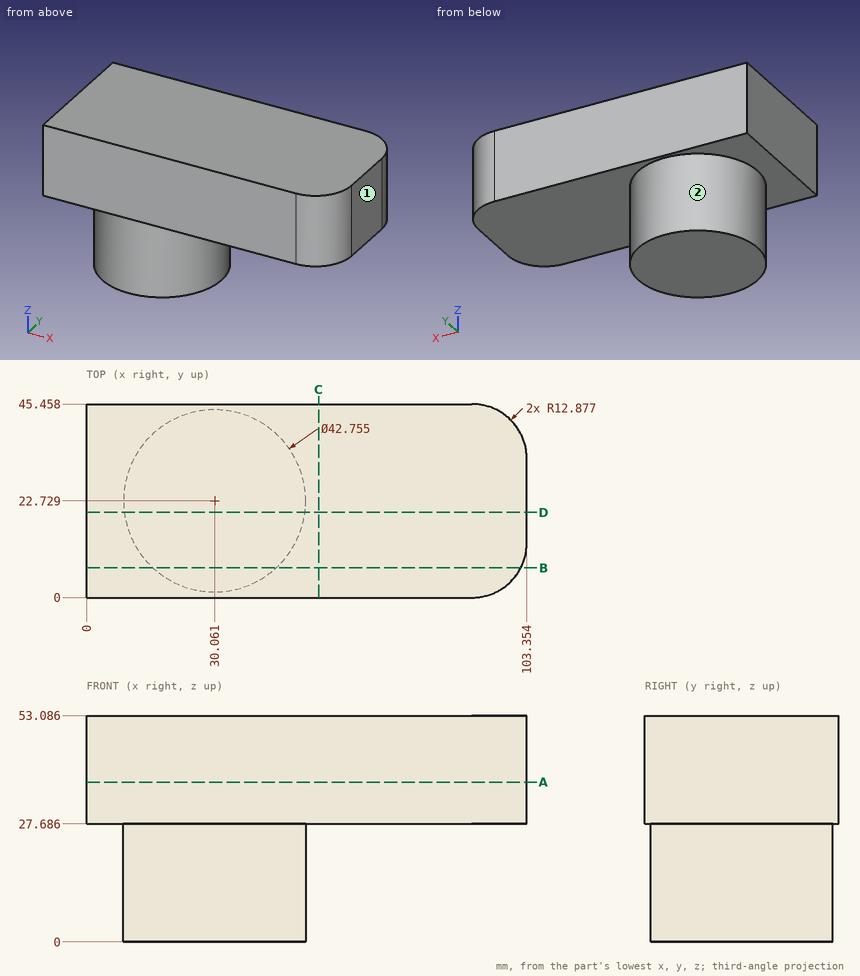
Here's the drawing with two shaded views (mm, measured from the low corner). I have some questions. A direction names the side the tool comes from. Give positions to 0.01 mm unless a question says otherwise; leave off trailing zeros. Loops run counter-clockwise (first coordinate to the right, second up) from the corner with the lowest first, then second, coordinate; pieces in that order, holes last. Notation, with made-up numbers: M 21,29 L 78,29 A16 cw 78,52 Z; hole C 52,83.25 d11. An arc over 180 degrees is marked long. Answer in a Markdown table with one row per item.
1. Suppose I cut it at C-C on x = 54.5. Write out the boundary of the cut face in (y, z).
Taken from the geometry:
| item | result |
|---|---|
| outline | M 0,27.69 L 45.46,27.69 L 45.46,53.09 L 0,53.09 Z |
2. Suppose I cut it at A-A on z = 37.5. Write out the boundary of the cut face in (x, y) (1 decimal).
Taken from the geometry:
| item | result |
|---|---|
| outline | M 0,0 L 90.5,0 A12.9 ccw 103.4,12.9 L 103.4,32.6 A12.9 ccw 90.5,45.5 L 0,45.5 Z |
3. Which directions (+Z, -Z, +X, -X, +Y, -Y) give clear straight access to the entire face, cutting with the end or side of a thin tool? Please do the marked faces 1 and 2.
Taken from the geometry:
| item | result |
|---|---|
| face 1 | +Z, -Z, +X, +Y, -Y |
| face 2 | -Z |
4. Suppose I cut it at D-D on y = 20. Write out the boundary of the cut face in (x, z).
Taken from the geometry:
| item | result |
|---|---|
| outline | M 0,27.69 L 8.86,27.69 L 8.86,0 L 51.26,0 L 51.26,27.69 L 103.35,27.69 L 103.35,53.09 L 0,53.09 Z |
5. Suppose I cut it at B-B on y = 7. Write out the boundary of the cut face in (x, z) (1 decimal).
Taken from the geometry:
| item | result |
|---|---|
| outline | M 0,27.7 L 15.6,27.7 L 15.6,0 L 44.5,0 L 44.5,27.7 L 101.9,27.7 L 101.9,53.1 L 0,53.1 Z |
6. For pin 1 Ø10 at (y, z) = (36.5, 42) entering from +X; pin 2 Ø1.5 at (y, z) = (10.5, 45.5) entering from +X; pin 3 Ø5 at (y, z) = (7.5, 24) entering from +X (1 decimal); pin 4 Ø1 at (x, y) = (49.5, 11) entering from -Z, each with a flat end and sliding along its axis, tell me the tip position at first contact or that it passes through.
Taken from the geometry:
| item | result |
|---|---|
| pin 1 | stops at x = 103.35 |
| pin 2 | stops at x = 103.25 |
| pin 3 | stops at x = 47.2 |
| pin 4 | stops at z = 27.69 |
7. If I drill on line 1 along Z through (x, y) = (77, 13.5); line 2 along Y through (x, z) = (31, 4) (1 decimal); line 3 along X through (y, z) = (4.5, 44.5) (1 decimal), over which ranges is the centre line in solid material (lowest first)?
Taken from the geometry:
| item | result |
|---|---|
| line 1 | z = 27.69 to 53.09 |
| line 2 | y = 1.4 to 44.1 |
| line 3 | x = 0 to 100.3 |
